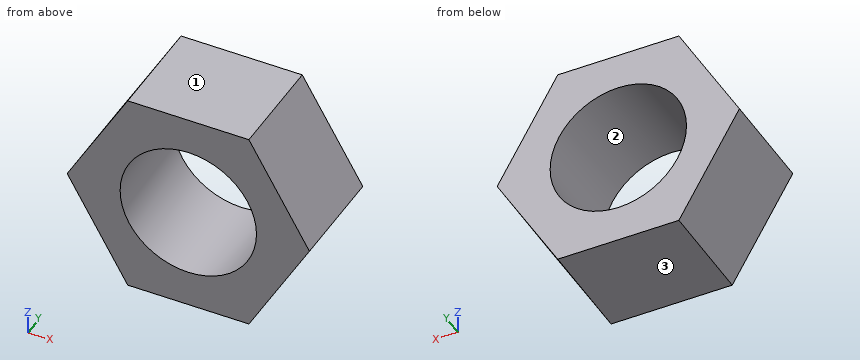
Autodesk Inventor part; units mm, degrees
ref_plane "YZ Plane" through (0, 0, 0) normal (1, 0, 0) x (0, 1, 0)
ref_plane "XZ Plane" through (0, 0, 0) normal (0, 1, 0) x (-1, 0, 0)
ref_plane "XY Plane" through (0, 0, 0) normal (0, 0, 1) x (1, 0, 0)
sketch "Sketch1" plane through (0, 0, 0) normal (0, 1, 0) x (-1, 0, 0)
  line L0 (6.6675, -3.8495) -> (8.89, 0)
  line L1 (6.6675, -3.8495) -> (2.2225, -3.8495)
  line L2 (2.2225, -3.8495) -> (0, 0)
  line L3 (6.6675, 3.8495) -> (8.89, 0)
  line L4 (6.6675, 3.8495) -> (2.2225, 3.8495)
  line L5 (2.2225, 3.8495) -> (0, 0)
  circle A0 centre (4.445, 0) radius 2.5019
  dimension "d5" = 5.0038
extrude "Extrusion1" add sketch "Sketch1" along normal blind 3.81
thread "Thread1"
properties part number "nut"
Model file for the job. Use its own axes, mm. Face numbers are marked on the shaded views. Give positions to 0.01 mm unless a question says otherwise; leave off trailing zeros. Order: outer loops, then holes, each group sorted by start corner. A loop starts at its lowest first (then second) coordinate and runs counter-clockwise, first axis right, second up. Notation, with made-up numbers: (29.5, 5.25) -> (44.5, 5.25) arc R16 ccw to (44.5, 36.25) -> close; hole circle Ø5 at (12.25, 2). An arc over 180 degrees is marked (long way). Use CSV: the item, a comma, the result in double quotes.
1. Band-saw the part on D-D, the plane z = 3.75. Give the cut face in (x, y), then the cut area to 3 significant figures.
Outcome:
outline,"(-6.72, 0) -> (-2.17, 0) -> (-2.17, 3.81) -> (-6.72, 3.81) -> close"
area,"17.4 mm²"
2. Drop a flat-ended pin along its axis: pin 1 (4 mm diameter, centred on x = -3.5, z = 1.5, fed in from -Y). Give the stop position or say it passes through.
Outcome:
pin 1,"y = 0"
3. Band-saw the part on B-B, the plane z = -1. Give the cut face in (x, y), then the cut area to 3 significant figures.
Outcome:
outline,"(-8.31, 0) -> (-6.74, 0) -> (-6.74, 3.81) -> (-8.31, 3.81) -> close; (-2.15, 0) -> (-0.58, 0) -> (-0.58, 3.81) -> (-2.15, 3.81) -> close"
area,"12.0 mm²"
4. Band-saw the part on C-C, the plane x = -3.75. Give the cut face in (y, z), then the cut area to 3 significant figures.
Outcome:
outline,"(0, -3.85) -> (3.81, -3.85) -> (3.81, -2.4) -> (0, -2.4) -> close; (0, 2.4) -> (3.81, 2.4) -> (3.81, 3.85) -> (0, 3.85) -> close"
area,"11.0 mm²"
5. Drill centre lines: line 1 along X through (y, z) = (0.2, -1.25); line 2 along Z through (x, y) = (-3.5, 0.4); line 3 along Z through (x, y) = (-6.75, 1.35). Where is each one in solid material? Low to high. Write a range as from..to.
Outcome:
line 1,"-8.17..-6.61, -2.28..-0.72"
line 2,"-3.85..-2.32, 2.32..3.85"
line 3,"-3.71..-0.97, 0.97..3.71"
6. Mould opens along Z. For the marked faces 1, 2 and 3 say: +Z half, -Z half, draft (parallel to the pull), parting line (faces both ways), or undercut.
Outcome:
face 1,"+Z half"
face 2,"undercut"
face 3,"-Z half"
7. Band-saw the part on A-A, the plane y = 3.25. Give the cut face in (x, z) (1 decimal), then the cut area to 3 significant figures.
Outcome:
outline,"(-8.9, 0) -> (-6.7, -3.8) -> (-2.2, -3.8) -> (0, 0) -> (-2.2, 3.8) -> (-6.7, 3.8) -> close; hole circle Ø5 at (-4.4, 0)"
area,"31.7 mm²"
